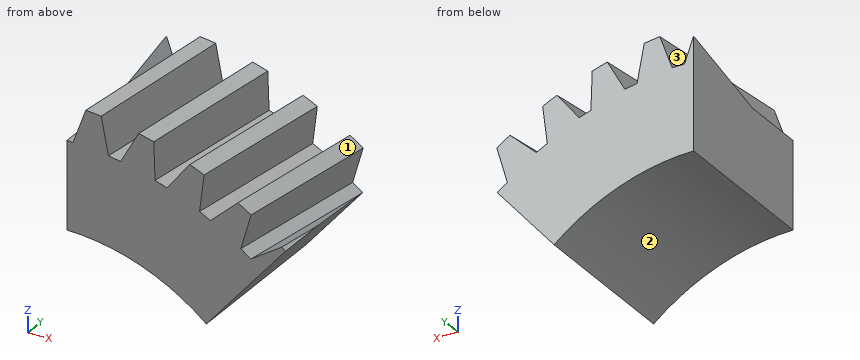
from build123d import *

# Parameters (mm, degrees)
SKETCH_1_R               = 31.5
SKETCH_1_R_2             = 20.1
EXTRUDE_1_DEPTH          = 15
PATTERN_CIRCULAR_4_COUNT = 40
SKETCH_9_OUTSIDE_W       = 83.064
SKETCH_9_OUTSIDE_H       = 83.064
CUT_EXTRUDE_1_DEPTH      = 48.00244519


with BuildPart() as part:
    # Эскиз1 → Бобышка-Вытянуть1 (new body)
    with BuildSketch(Plane(origin=(0, 0, 0), x_dir=(1, 0, 0), z_dir=(0, 1, 0))):
        with Locations(Location((0, 0, 0), (0, 0, 270))):
            Circle(SKETCH_1_R)
        with Locations(Location((0, 0, 0), (0, 0, 270))):
            Circle(SKETCH_1_R_2, mode=Mode.SUBTRACT)
    extrude(amount=EXTRUDE_1_DEPTH)

    # Вырез-По траектории4: sweep along a path in Эскиз8
    with BuildLine(Plane(origin=(30, 0, 0), x_dir=(0, 0, -1), z_dir=(1, 0, 0))) as sweep_4_path:
        Line((0, 0), (1.610154635, 17.19379209))
    # Эскиз7 → Вырез-По траектории4 (sweep, cut)
    with BuildSketch(Plane(origin=(0, 0, 0), x_dir=(1, 0, 0), z_dir=(0, 1, 0))):
        Polygon((28.2, -0.57191311), (28.2, 0.57191311), (32, 1.955), (32, -1.955), align=None)
    sweep_4 = sweep(path=sweep_4_path.line, mode=Mode.SUBTRACT)

    # Круговой массив4: Вырез-По траектории4 ×40 about axis
    pattern_circular_4_axis = Axis((0, 0, 0), (0, 1, 0))
    for i in range(1, PATTERN_CIRCULAR_4_COUNT):
        add(sweep_4.rotate(pattern_circular_4_axis, i * 360 / PATTERN_CIRCULAR_4_COUNT), mode=Mode.SUBTRACT)

    # Эскиз9 outside → Вырез-Вытянуть1 (cut, through all)
    with BuildSketch(Plane(origin=(0, 15, 0), x_dir=(1, 0, 0), z_dir=(0, 1, 0))):
        Rectangle(SKETCH_9_OUTSIDE_W, SKETCH_9_OUTSIDE_H)
        with BuildLine():
            Line((0, 0), (0, -31.5))
            ThreePointArc((0, -31.5), (10.773634515, -29.600317555), (20.247809705, -24.130399958))
            Line((20.247809705, -24.130399958), (0, 0))
        make_face(mode=Mode.SUBTRACT)
    extrude(amount=-CUT_EXTRUDE_1_DEPTH, mode=Mode.SUBTRACT)


solid = part.part
Work out the finished part from the listing and answer in its coordinate system (mm). Face numbers are marked on the shaded views. Round coordinates to 2 decimals unless told otherwise and drop trailing zeros. Write each loop counter-clockwise with the first axis right and the second up, starting at its lowest first coordinate (ties: lowest second). Pieces come first, ordered by that corner, then holes. Notation, with made-up numbers: M -19,66 L 39,66 A19 ccw 39,96 Z; hole C -33.5,66.5 d3. An arc over 180 degrees is marked long. Use a Markdown table: item, result.
1) The part is cut by section C-C on z = 21. Give the vertices of the cut face in (x, y).
Taken from the geometry:
| item | result |
|---|---|
| outline | M 0,0 L 17.62,0 L 17.62,15 L 0,15 Z |
2) The part is cut by section B-B on y = 8. Give the vertices of the cut face in (x, z), plus the area to 3 significant figures.
Taken from the geometry:
| item | result |
|---|---|
| outline | M 0,20.1 A20.1 cw 12.92,15.4 L 19.6,23.35 L 17.64,22.04 L 16.72,22.71 L 17.68,26.07 A31.5 ccw 16.47,26.85 L 13.98,24.53 L 12.96,25.05 L 13.39,28.51 A31.5 ccw 12.07,29.1 L 9.97,26.41 L 8.88,26.77 L 8.76,30.26 A31.5 ccw 7.37,30.63 L 5.72,27.65 L 4.59,27.83 L 3.92,31.26 A31.5 ccw 2.49,31.4 L 1.32,28.2 L 0.18,28.2 L 0,28.69 Z |
| area | 169 mm2 |
3) Consider line 1 (X direction, y = 12.75, z = 29); line 2 (X direction, y = 4.25, z = 30); line 3 (X direction, y = 6.25, z = 18). Determine where each line is inside the solid, lowest interval first. Write a range as [from, to].
Taken from the geometry:
| item | result |
|---|---|
| line 1 | x = [0, 0.33], [2.06, 4.78], [6.94, 9.22] |
| line 2 | x = [1.63, 3.83], [6.64, 8.44] |
| line 3 | x = [8.94, 15.1] |
4) The part is cut by section A-A on x = 17.5. Give the vertices of the cut face in (y, z), plus the area to 3 significant figures.
Taken from the geometry:
| item | result |
|---|---|
| outline | M 0,20.86 L 15,20.86 L 15,22.14 L 6.09,22.14 L 0,22.79 Z; M 5.63,26.19 L 15,23.2 L 15,26.19 Z |
| area | 35.3 mm2 |
5) Determine the mould class of the marked faces 1, 2 and 3 for opening direction X: pulls with the +X half, pulls with the -X half, needs draft (parallel to the pull), parting line crosses it, or undercut.
Taken from the geometry:
| item | result |
|---|---|
| face 1 | pulls with the +X half |
| face 2 | pulls with the -X half |
| face 3 | undercut |
6) Flat-ended cylindrical pins translate along their axes: pin 1 (1.5 mm diameter, centred on y = 9.5, z = 17.5, fed in from +X); pin 2 (6 mm diameter, centred on x = 3, y = 4, fed in from -Z); pin 3 (1 mm diameter, centred on x = 7, z = 26.5, fed in from -Y); pin 4 (6 mm diameter, centred on x = 16, y = 11, fed in from +Z). Find the tip coordinate at first contact, or state that the pin passes through.
Taken from the geometry:
| item | result |
|---|---|
| pin 1 | stops at x = 15.31 |
| pin 2 | stops at z = 19.18 |
| pin 3 | stops at y = 0 |
| pin 4 | stops at z = 28.69 |
7) The part is cut by section D-D on x = 9. Give the vertices of the cut face in (y, z).
Taken from the geometry:
| item | result |
|---|---|
| outline | M 0,17.97 L 15,17.97 L 15,30.19 L 10.69,30.19 L 9.32,26.73 L 0,26.73 Z |
